Design review of the part built by this model. Coordinates are the model's own, in mm. A direction names the side the tool comes from. Give positions to 0.01 mm unless a question says otherwise; leave off trailing zeros. Write each loop counter-clockwise with the first axis right and the second up, starting at its lowest first coordinate (ties: lowest second). Pieces come first, ordered by that corner, then holes. Notation, with made-up numbers: (29, -32.75) -> (54, -32.75) arc R25 cw to (54, -8.75) -> close; hole circle Ø3 at (25.25, 51.5). An arc over 180 degrees is marked (long way). Return JSON: item names as keys, results as strings. Group by question number.
from build123d import *

# Parameters (mm, degrees)
F0_R     = 107.95
F1_DEPTH = 25.4
F2_R     = 38.1
F3_DEPTH = 304.8
F4_W     = 25.4
F4_H     = 25.4
F5_DEPTH = 203.2


with BuildPart() as f1:
    # F0 (on Top) → F1 (new body)
    with BuildSketch(Plane.XY):
        Circle(F0_R)
    extrude(amount=F1_DEPTH)

    # F2 (on face) → F3 (join)
    with BuildSketch(Plane.XY.offset(25.4)):
        Circle(F2_R)
    extrude(amount=F3_DEPTH)

    # F4 (on Right) → F5 (join)
    with BuildSketch(Plane.YZ):
        with Locations((0, 165.1)):
            Rectangle(F4_W, F4_H)
    extrude(amount=F5_DEPTH)


solid = f1.part
Q1. Insertion check: pin 1 (20.5 mm diameter, centred on x = 152.5, z = 162, fed in from -Y); pin 2 (4 mm diameter, centred on x = 19.5, y = 37, fed in from +Z); pin 3 (20.5 mm diameter, centred on x = 82.5, z = 163.5, fed in from +Y). Each pin has a flat end and moves straight along its axis. Give the tip position at first contact, or say it passes through.
Q2. Take a section at C-C, the plane x = 0. Give the boundary of the cut face in (y, z), plus the area to 3 significant figures.
Q3. Tool access review of faces 1 (the face through (-2, 2, 0)), 2 (the face through (118, 12.7, 165)), 3 (the face through (118, -12.7, 165)): name each direction out of +Z, -Z, +X, -X, +Y, -Y from which nothing blocks a thin tool from reaching the whole face with its end or side.
Q4. For L1, parallel to Z at x = 48, y = 40; L2, parallel to Y at x = 126, z = 175; L3, parallel to X at y = 17, z = 250.5, list the stretches that pass through material, from the lowest coordinate up. Write a range as from..to.
Q5. Take a section at D-D, the plane z = 45. Give the boundary of the cut face in (x, y).
Q6. Take a section at B-B, the plane y = 0. Give the boundary of the cut face in (x, z).
Q7. Take a section at A-A, the plane x = 95.5. Give the boundary of the cut face in (y, z).
Final values:
{
 "1": {"pin 1": "stops at y = -12.7", "pin 2": "stops at z = 25.4", "pin 3": "stops at y = 12.7"},
 "2": {"outline": "(-107.95, 0) -> (107.95, 0) -> (107.95, 25.4) -> (38.1, 25.4) -> (38.1, 330.2) -> (-38.1, 330.2) -> (-38.1, 25.4) -> (-107.95, 25.4) -> close", "area": "28,700 mm²"},
 "3": {"face 1": "-Z, +X, -X, +Y, -Y", "face 2": "+Z, +X, +Y", "face 3": "+Z, +X, -Y"},
 "4": {"L1": "z = 0..25.4", "L2": "y = -12.7..12.7", "L3": "x = -34.1..34.1"},
 "5": {"outline": "circle Ø76.2 at (0, 0)"},
 "6": {"outline": "(-107.95, 0) -> (107.95, 0) -> (107.95, 25.4) -> (38.1, 25.4) -> (38.1, 152.4) -> (203.2, 152.4) -> (203.2, 177.8) -> (38.1, 177.8) -> (38.1, 330.2) -> (-38.1, 330.2) -> (-38.1, 25.4) -> (-107.95, 25.4) -> close"},
 "7": {"outline": "(-50.33, 0) -> (50.33, 0) -> (50.33, 25.4) -> (-50.33, 25.4) -> close; (-12.7, 152.4) -> (12.7, 152.4) -> (12.7, 177.8) -> (-12.7, 177.8) -> close"}
}
